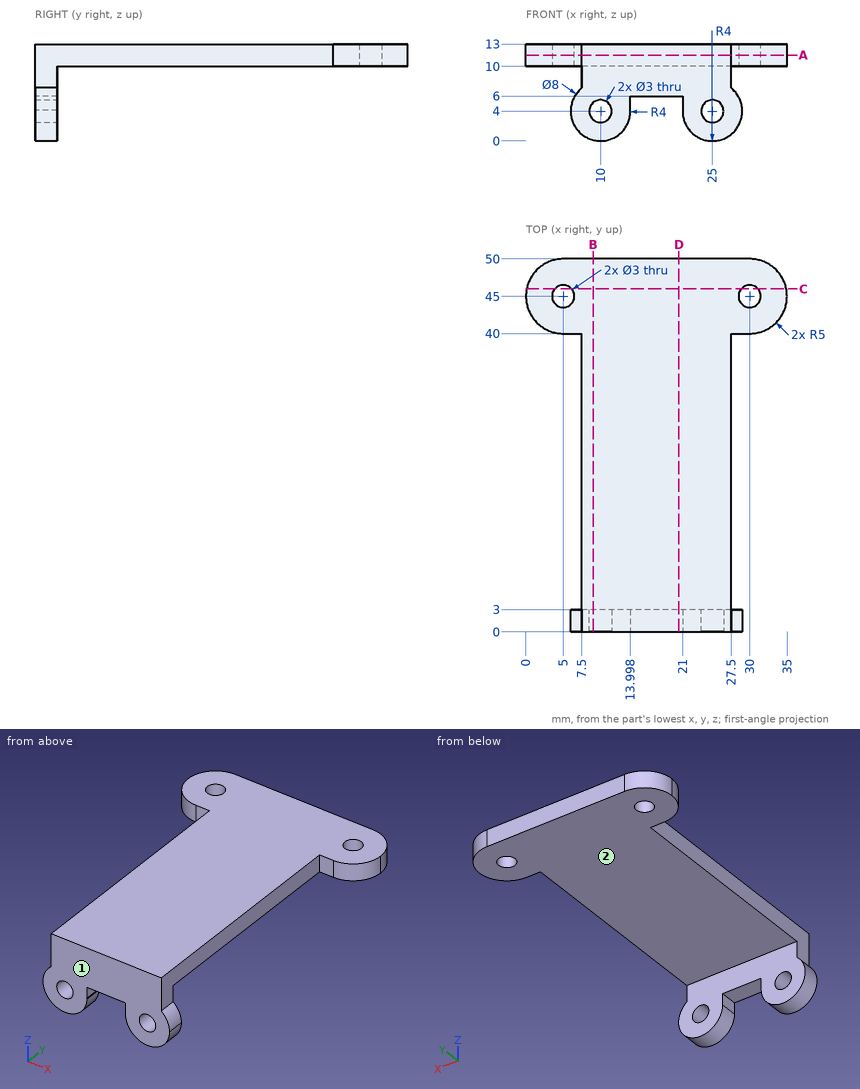
Study the drawing (mm; zero at the part's minimum x, y, z) and answer. A direction names the side the tool comes from. Round coordinates to 2 decimals unless told otherwise and drop trailing zeros. Loops run counter-clockwise (first coordinate to the right, second up) from the corner with the lowest first, then second, coordinate; pieces in that order, holes last. Notation, with made-up numbers: (70.5, 70) -> (83.5, 70) arc R20 cw to (83.5, 104) -> close; hole circle Ø11 at (-23.5, 39). An arc over 180 degrees is marked (long way). Write each question's results on one line, items separated by ' | '. Start each with the question number.
1. Section C-C (y = 46) is taken. Determine the outline of the cut face in (x, z).
2. Section B-B (x = 9) is taken. Determine the outline of the cut face in (y, z), plus the area to 3 significant figures.
3. Section D-D (x = 20.5) is taken. Determine the outline of the cut face in (y, z).
4. Section A-A (z = 11.5) is taken. Determine the outline of the cut face in (x, y), plus the area to 3 significant figures.
5. Given pin 1 Ø12 at (x, y) = (7.5, 42.5) entering from -Z; pin 2 Ø5 at (x, z) = (25, 4) entering from +Y; pin 3 Ø2 at (y, z) = (2, 5) entering from +X; pin 4 Ø1.8 at (y, z) = (21.5, 9) entering from -X, each flat-ended and moving along its own axis, determine where each tip first touches the part or whether it passes through.
6. Find the intervals of material crossed by probe 1 along Z at (x, y) = (10, 2.3); probe 2 along Z at (x, y) = (16.5, 45.5); probe 3 along X at (y, z) = (30, 10.75), in increasing order. Write a range as from..to.
7. A tool of negligible diameter and unlimited length cuts with its end or side. For the marked faces 1 and 2, from which of +Z, -Z, +X, -X, +Y, -Y can it reach the whole face along a straight path? Write none if from no direction.
Evaluation:
1) outline: (0.1, 10) -> (3.88, 10) -> (3.88, 13) -> (0.1, 13) -> close; (6.12, 10) -> (28.88, 10) -> (28.88, 13) -> (6.12, 13) -> close; (31.12, 10) -> (34.9, 10) -> (34.9, 13) -> (31.12, 13) -> close
2) outline: (0, 0.13) -> (3, 0.13) -> (3, 2.88) -> (0, 2.88) -> close; (0, 5.12) -> (3, 5.12) -> (3, 10) -> (50, 10) -> (50, 13) -> (0, 13) -> close | area: 173 mm2
3) outline: (0, 6) -> (3, 6) -> (3, 10) -> (50, 10) -> (50, 13) -> (0, 13) -> close
4) outline: (5, 40) -> (7.5, 40) -> (7.5, 0) -> (27.5, 0) -> (27.5, 40) -> (30, 40) arc R5 ccw to (30, 50) -> (5, 50) arc R5 ccw to start; hole circle Ø3 at (5, 45); hole circle Ø3 at (30, 45) | area: 1,110 mm2
5) pin 1: stops at z = 10 | pin 2: stops at y = 3 | pin 3: stops at x = 29 | pin 4: passes through
6) probe 1: z = 0..2.5, 5.5..13 | probe 2: z = 10..13 | probe 3: x = 7.5..27.5
7) face 1: +Z, -Z, +X, -X, -Y | face 2: -Z, +X, -X, +Y
